The model under review builds one solid part; all positions refer to its coordinate system, in mm. Face numbers are marked on the shaded views. A direction names the side the tool comes from. Coordinates: 2 decimals unless noted, no trailing zeros. Loops run counter-clockwise (first coordinate to the right, second up) from the corner with the lowest first, then second, coordinate; pieces in that order, holes last. Notation, with made-up numbers: (61.25, -39) - (97.25, -39) arc R22 cw to (97.25, -26) - close; hole circle Ø10 at (-36, -21.5). An arc over 180 degrees is marked (long way). Answer in a Markdown table with one row per item. Add a question column.
(1) We need section B-B on x = -5. Write out the cut boundary in (y, z), plus the area to 3 significant figures.
(2) We need section D-D on z = 6.5. Write out the cut boundary in (x, y).
(3) For line 1 along Y through (x, z) = (104.5, 7.25); line 2 along Y through (x, z) = (62, 7); line 3 along X through (y, z) = (104, 5), list the stretches that pass through material, from the lowest coordinate up.
(4) We need section C-C on x = 62. Write out the cut boundary in (y, z), plus the area to 3 significant figures.
(5) For P1, Ø5, axis at x = 54, z = 8, coming from the +Y side; P2, Ø5, axis at y = 88.5, z = 6, coming from the -X side; P3, Ø6, axis at x = 59, y = 115.5, coming from the +Z side, all flat-tipped, find the tip position at first contact; note any pin that passes through.
(6) Machinability: for the marked faces 1 and 2, which of the approach directions +Z, -Z, +X, -X, +Y, -Y give a long, thin tool a straight path to every point of the face, cutting with its end or side? Answer none if there is none.
(7) We need section A-A on y = 62. Write out the cut boundary in (x, z), plus the area to 4 significant figures.
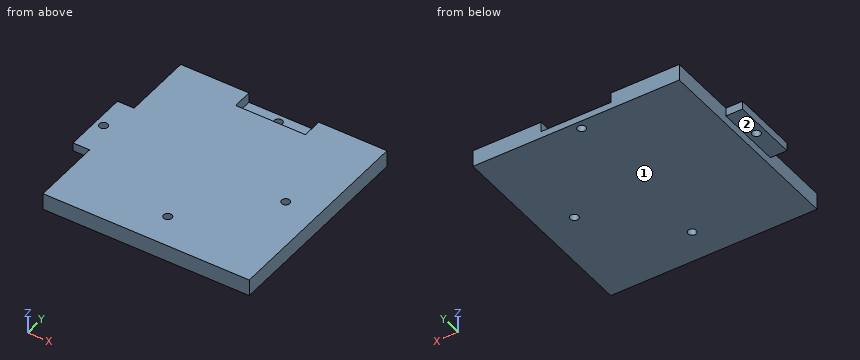
Autodesk Inventor part; units mm, degrees
ref_plane "YZ Plane" through (0, 0, 0) normal (1, 0, 0) x (0, 1, 0)
ref_plane "XZ Plane" through (0, 0, 0) normal (0, 1, 0) x (-1, 0, 0)
ref_plane "XY Plane" through (0, 0, 0) normal (0, 0, 1) x (1, 0, 0)
sketch "Sketch1" plane through (0, 0, 0) normal (0, 0, 1) x (1, 0, 0)
  line L0 (0, 0) -> (124, 0)
  line L1 (124, 0) -> (124, 124)
  line L2 (124, 124) -> (0, 124)
  line L3 (0, 124) -> (0, 0)
  dimension "d0" = 124
  dimension "d1" = 124
extrude "Extrusion1" add sketch "Sketch1" along normal blind 10
sketch "Sketch2" plane through (0, 0, 10) normal (0, 0, 1) x (1, 0, 0)
  line L0 (124, 124) -> (0, 124)
  line L1 (41, 124) -> (83, 124)
  line L2 (83, 124) -> (83, 112)
  line L3 (83, 112) -> (41, 112)
  line L4 (41, 112) -> (41, 124)
  point P0 (0, 0)
  point P1 (62, 112)
  point P2 (62, 124)
  dimension "d4" = 42
  dimension "d5" = 12
extrude "Extrusion2" cut sketch "Sketch2" against normal blind 6
sketch "Sketch3" plane through (0, 0, 4) normal (0, 0, 1) x (1, 0, 0)
  circle A0 centre (62, 119) radius 2.5
  line L0 (41, 124) -> (83, 124) construction
  line L1 (41, 112) -> (41, 124) construction
  line L2 (83, 112) -> (41, 112) construction
  line L3 (83, 124) -> (83, 112) construction
  point P0 (0, 0)
  point P1 (62, 124)
  point P2 (83, 118)
  dimension "d8" = 5
  dimension "d22" = 5
extrude "Extrusion3" cut sketch "Sketch3" against normal through all
sketch "Sketch4" plane through (0, 0, 10) normal (0, 0, 1) x (1, 0, 0)
  line L0 (0, 124) -> (0, 0)
  line L1 (0, 82) -> (-10, 82)
  line L2 (-10, 82) -> (-10, 42)
  line L3 (-10, 42) -> (0, 42)
  line L4 (0, 42) -> (0, 82)
  circle A0 centre (-5, 62) radius 2.5
  point P0 (-10, 62)
  point P1 (0, 62)
  point P2 (-5, 82)
  dimension "d11" = 10
  dimension "d12" = 40
  dimension "d13" = 5
extrude "Extrusion4" add sketch "Sketch4" against normal blind 5
sketch "Sketch5" plane through (0, 0, 10) normal (0, 0, 1) x (1, 0, 0)
  circle A0 centre (62, 19.5) radius 2.5
  line L0 (0, 0) -> (124, 0)
  circle A1 centre (104.5, 62) radius 2.5
  line L1 (124, 0) -> (124, 124)
  point P0 (62, 0)
  point P1 (124, 62)
  dimension "d16" = 5
  dimension "d17" = 19.5
  dimension "d18" = 5
  dimension "d19" = 19.5
extrude "Extrusion5" cut sketch "Sketch5" against normal through all
properties part number "TC001" material "ABS Plastic"
Outcome:
| question | item | result |
|---|---|---|
| 1 | outline | (42, 5) - (59.5, 5) - (59.5, 10) - (42, 10) - close; (64.5, 5) - (82, 5) - (82, 10) - (64.5, 10) - close |
| 1 | area | 175 mm² |
| 2 | outline | (-10, 42) - (0, 42) - (0, 0) - (124, 0) - (124, 124) - (83, 124) - (83, 112) - (41, 112) - (41, 124) - (0, 124) - (0, 82) - (-10, 82) - close; hole circle Ø5 at (-5, 62); hole circle Ø5 at (62, 19.5); hole circle Ø5 at (104.5, 62) |
| 3 | line 1 | 0 to 59.5, 64.5 to 124 |
| 3 | line 2 | 0 to 17, 22 to 112 |
| 3 | line 3 | 0 to 124 |
| 4 | outline | (0, 0) - (17, 0) - (17, 10) - (0, 10) - close; (22, 0) - (116.5, 0) - (116.5, 4) - (112, 4) - (112, 10) - (22, 10) - close; (121.5, 0) - (124, 0) - (124, 4) - (121.5, 4) - close |
| 4 | area | 1,100 mm² |
| 5 | P1 | y = 112 |
| 5 | P2 | x = 0 |
| 5 | P3 | z = 4 |
| 6 | face 1 | -Z, +X, -X, +Y, -Y |
| 6 | face 2 | -Z, -X, +Y, -Y |
| 7 | outline | (-10, 5) - (-7.5, 5) - (-7.5, 10) - (-10, 10) - close; (-2.5, 5) - (0, 5) - (0, 0) - (102, 0) - (102, 10) - (-2.5, 10) - close; (107, 0) - (124, 0) - (124, 10) - (107, 10) - close |
| 7 | area | 1,215 mm² |
